For this review, use the dimensioned drawing (mm, ordinates from the lowest corner) and the shaded views. A direction names the side the tool comes from. Coordinates: 2 decimals unless noted, no trailing zeros. Loops run counter-clockwise (first coordinate to the right, second up) from the corner with the lowest first, then second, coordinate; pieces in that order, holes last. Notation, with made-up numbers: M 41.5,71 L 58.5,71 A19 ccw 58.5,106 Z; hole C -39,42 d11. An arc over 180 degrees is marked long. Write item = value, one per line.
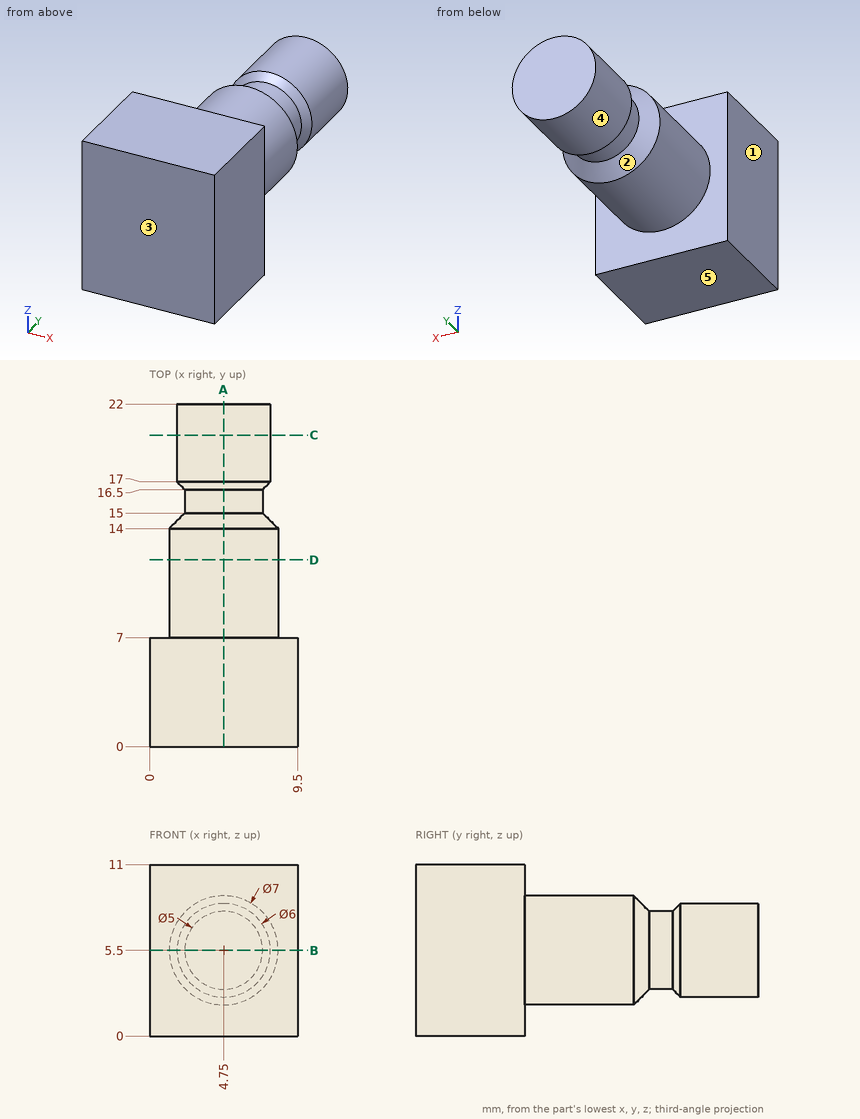
Q1. For line 1 along Y through (x, z) = (5.5, 1); line 2 along X through (y, z) = (16.75, 4); line 3 along Z through (x, y) = (6, 12), list the stretches that pass through material, from the lowest coordinate up.
Solved:
line_1 = 0 to 7
line_2 = 2.45 to 7.05
line_3 = 2.23 to 8.77
Q2. Draft analysis for pull direction Y (two halves, no side actions). For the marked faces 1, 2 and 3, state which applies: +Y half, -Y half, draft (parallel to the pull), parting line (faces both ways), or undercut.
Solved:
face_1 = draft
face_2 = undercut
face_3 = -Y half
Q3. Add section A-A (x = 4.75). Write out the cut boundary in (y, z), and give its area (3 significant figures).
Solved:
outline = M 0,0 L 7,0 L 7,2 L 14,2 L 15,3 L 16.5,3 L 17,2.5 L 22,2.5 L 22,8.5 L 17,8.5 L 16.5,8 L 15,8 L 14,9 L 7,9 L 7,11 L 0,11 Z
area = 172 mm²
Q4. Machinability: for the marked faces 4 and 5, which of the approach directions +Z, -Z, +X, -X, +Y, -Y give a long, thin tool a straight path to every point of the face, cutting with its end or side? Answer none if there is none.
Solved:
face_4 = +Y
face_5 = -Z, +X, -X, +Y, -Y
Q5. Add section C-C (y = 20). Write out the cut boundary in (x, z), and give its area (3 significant figures).
Solved:
outline = C 4.75,5.5 d6
area = 28.3 mm²
Q6. For pin 1 Ø5 at (x, y) = (7.5, 13) entering from +Z; pin 2 Ø3 at (y, z) = (12, 9) entering from -X, all flat-tipped, find the tip position at first contact; note any pin that passes through.
Solved:
pin_1 = 8.99
pin_2 = 1.88
Q7. Add section B-B (z = 5.5). Write out the cut boundary in (x, y), and give its area (3 significant figures).
Solved:
outline = M 0,0 L 9.5,0 L 9.5,7 L 8.25,7 L 8.25,14 L 7.25,15 L 7.25,16.5 L 7.75,17 L 7.75,22 L 1.75,22 L 1.75,17 L 2.25,16.5 L 2.25,15 L 1.25,14 L 1.25,7 L 0,7 Z
area = 162 mm²
Q8. Add section D-D (y = 12). Write out the cut boundary in (x, z).
Solved:
outline = C 4.75,5.5 d7
